The listing builds one solid part. Answer for the finished solid, in the listing's coordinates (mm). A direction names the side the tool comes from. Coordinates: 2 decimals unless noted, no trailing zeros. Order: outer loops, then holes, each group sorted by start corner. A loop starts at its lowest first (then second) coordinate and runs counter-clockwise, first axis right, second up. Notation, with made-up numbers: (-30.5, -29) - (4.5, -29) arc R20 ccw to (4.5, -13) - close; hole circle Ø1 at (-14, 57). An arc over 180 degrees is marked (long way). One line per item, written item: value. Start each with the question number.
```python
from build123d import *

# Parameters (mm, degrees)
SKETCH1_R           = 9.6
BOSS_EXTRUDE1_DEPTH = 34
SKETCH2_R           = 2
CUT_EXTRUDE1_DEPTH  = 34
SKETCH3_R           = 4
CUT_EXTRUDE2_DEPTH  = 34
SKETCH4_R           = 9.6
SKETCH4_R_2         = 8.5
BOSS_EXTRUDE2_DEPTH = 2
CHAMFER1_SIZE       = 1


with BuildPart() as part:
    # Sketch1 → Boss-Extrude1 (new body)
    with BuildSketch(Plane.XY):
        with BuildLine():
            Line((16.733200531, 7), (22.5, 7))
            Line((22.5, 7), (22.5, 12))
            Line((22.5, 12), (-22.5, 12))
            Line((-22.5, 12), (-22.5, 7))
            Line((-22.5, 7), (-16.733200531, 7))
            ThreePointArc((-16.733200531, 7), (-13.665340575, 5.566755792), (-12.795976876, 2.294117647))
            ThreePointArc((-12.795976876, 2.294117647), (0, -13), (12.795976876, 2.294117647))
            ThreePointArc((12.795976876, 2.294117647), (13.665340575, 5.566755792), (16.733200531, 7))
        make_face()
        Circle(SKETCH1_R, mode=Mode.SUBTRACT)
    extrude(amount=BOSS_EXTRUDE1_DEPTH)

    # Sketch2 → Cut-Extrude1 (cut)
    with BuildSketch(Plane(origin=(0, 12, 0), x_dir=(1, 0, 0), z_dir=(0, 1, 0))):
        with Locations(Location((-18, -29.5, 0), (0, 0, 270))):  # turned: the seam where the file's is
            Circle(SKETCH2_R)
        with Locations(Location((18, -29.5, 0), (0, 0, 270))):  # turned: the seam where the file's is
            Circle(SKETCH2_R)
        with Locations(Location((18, -4.5, 0), (0, 0, 270))):  # turned: the seam where the file's is
            Circle(SKETCH2_R)
        with Locations(Location((-18, -4.5, 0), (0, 0, 270))):  # turned: the seam where the file's is
            Circle(SKETCH2_R)
    extrude(amount=-CUT_EXTRUDE1_DEPTH, mode=Mode.SUBTRACT)

    # Sketch3 → Cut-Extrude2 (cut)
    with BuildSketch(Plane.XZ.offset(-7)):
        with Locations((-18, 29.5)):
            Circle(SKETCH3_R)
        with Locations((-18, 4.5)):
            Circle(SKETCH3_R)
        with Locations((18, 4.5)):
            Circle(SKETCH3_R)
        with Locations((18, 29.5)):
            Circle(SKETCH3_R)
    extrude(amount=CUT_EXTRUDE2_DEPTH, mode=Mode.SUBTRACT)

    # Sketch4 → Boss-Extrude2 (add)
    with BuildSketch(Plane(origin=(0, 0, 0), x_dir=(-1, 0, 0), z_dir=(0, 0, -1))):
        Circle(SKETCH4_R)
        Circle(SKETCH4_R_2, mode=Mode.SUBTRACT)
    extrude(amount=-BOSS_EXTRUDE2_DEPTH)

    # Chamfer1
    chamfer1_edges = [part.edges().sort_by_distance(p)[0] for p in [
        (-9.6, 0, 34),
    ]]
    chamfer(chamfer1_edges, length=CHAMFER1_SIZE)


solid = part.part
```
(1) The part is cut by section C-C on z = 29.5. Determine the outline of the cut face in (x, y), plus the area to 3 significant figures.
(2) The part is cut by section B-B on x = 18. Determine the outline of the cut face in (y, z).
(3) The part is cut by section A-A on y = 0. Determine the outline of the cut face in (x, z).
(4) The part is cut by section D-D on z = 12. Determine the outline of the cut face in (x, y), plus the area to 3 significant figures.
(5) Consider probe 1 along Y at (x, z) = (0, 17); probe 2 along X at (y, z) = (10.85, 4.5); probe 3 along Y at (x, z) = (0, 0.9). Determine where each line is inside the solid, lowest interval first.
(6) Flat-ended cylindrical pins translate along their axes: pin 1 Ø3 at (y, z) = (-1, 18.5) entering from +X; pin 2 Ø3 at (x, z) = (18, 4.5) entering from +Y; pin 3 Ø5 at (x, z) = (17, 22) entering from -Y; pin 4 Ø1.5 at (y, z) = (-10, 14.5) entering from -X. Find the tip coordinate at first contact, or state that the pin passes through.
(7) For faces 4 (the face through (-14, 6.6, 4.4)), 5 (the face through (5.161, 8.095, 17.283)), 6 (the face through (14, 6.6, 29.6)), 7 (the face through (22.5, 9, 17)), determine the directions among +Z, -Z, +X, -X, +Y, -Y from which every point of the face is accessible in a straight line to the end or side of a thin tool.
(8) For a pull along Y with two mould halves and no side action, classify faces 1 (the face through (-2, 11, 34)), 2 (the face through (-4.57, 7.167, 0.986)), 3 (the face through (0, 12, 17)) as pulls with the +Y half, pulls with the -Y half, needs draft (parallel to the pull), parting line crosses it, or undercut.
Completed:
1. outline: (-22.5, 7) - (-20, 7) - (-20, 12) - (-22.5, 12) - close; (-16, 7) - (-14, 7) - (-14, 5.92) arc R4 cw to (-12.8, 2.29) arc R13 ccw (long way) to (12.8, 2.29) arc R4 cw to (14, 5.92) - (14, 7) - (16, 7) - (16, 12) - (-16, 12) - close; (20, 7) - (22.5, 7) - (22.5, 12) - (20, 12) - close; hole circle Ø19.2 at (0, 0)
1. area: 345 mm2
2. outline: (7, 0) - (12, 0) - (12, 2.5) - (7, 2.5) - close; (7, 6.5) - (12, 6.5) - (12, 27.5) - (7, 27.5) - close; (7, 31.5) - (12, 31.5) - (12, 34) - (7, 34) - close
3. outline: (-13, 0) - (-8.5, 0) - (-8.5, 2) - (-9.6, 2) - (-9.6, 33) - (-10.6, 34) - (-13, 34) - close; (8.5, 0) - (13, 0) - (13, 34) - (10.6, 34) - (9.6, 33) - (9.6, 2) - (8.5, 2) - close
4. outline: (-22.5, 7) - (-16.73, 7) arc R4 cw to (-12.8, 2.29) arc R13 ccw (long way) to (12.8, 2.29) arc R4 cw to (16.73, 7) - (22.5, 7) - (22.5, 12) - (-22.5, 12) - close; hole circle Ø19.2 at (0, 0)
4. area: 387 mm2
5. probe 1: y = -13 to -9.6, 9.6 to 12
5. probe 2: x = -22.5 to -20, -16 to 16, 20 to 22.5
5. probe 3: y = -13 to -8.5, 8.5 to 12
6. pin 1: stops at x = 13
6. pin 2: passes through
6. pin 3: stops at y = 6.32
6. pin 4: stops at x = -9.13
7. face 4: -X, -Y
7. face 5: +Z
7. face 6: +X, -Y
7. face 7: +Z, -Z, +X, +Y, -Y
8. face 1: needs draft
8. face 2: undercut
8. face 3: pulls with the +Y half
